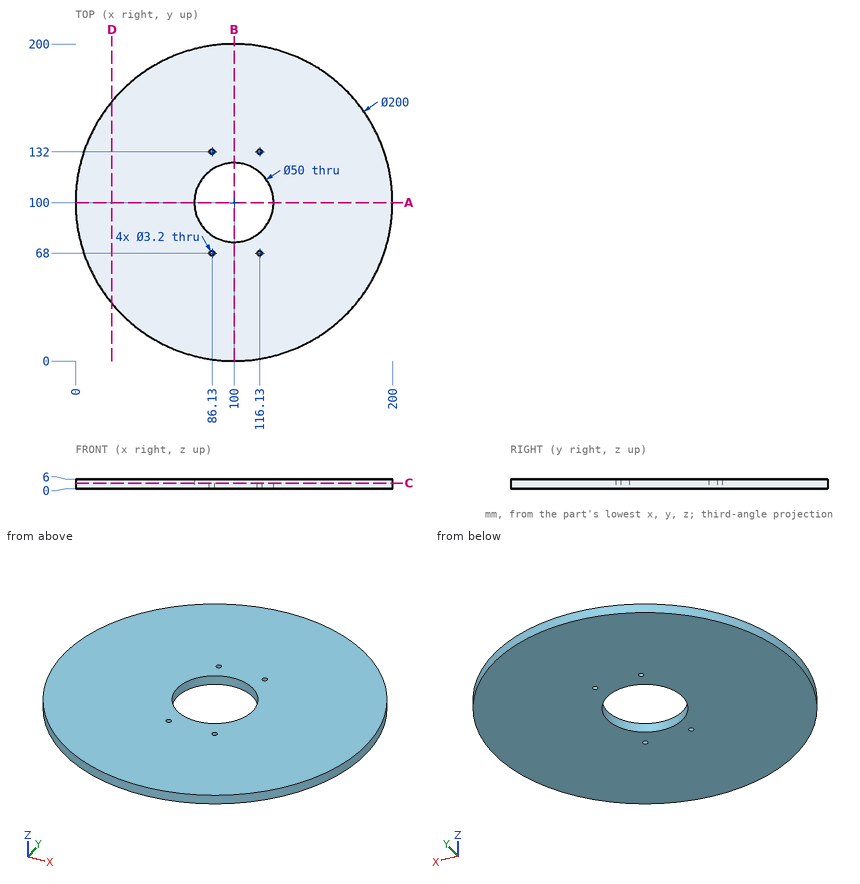
Print and shaded views of the part. All mm, measured from the part's lowest x, y and z. Give positions to 0.01 mm unless a question says otherwise; leave off trailing zeros. Write each loop counter-clockwise with the first axis right and the second up, starting at its lowest first coordinate (ties: lowest second). Pieces come first, ordered by that corner, then holes. Notation, with made-up numbers: (-22.75, -32.75) -> (-14.75, -32.75) arc R25 ccw to (-14.75, 1.25) -> close; hole circle Ø8 at (-15, 68.25). An arc over 180 degrees is marked (long way). Write item = value, one per line.
(1) Slice it at C-C, the plane z = 3.45. Give the cut face in (x, y).
Determined:
outline = circle Ø200 at (100, 100); hole circle Ø50 at (100, 100); hole circle Ø3.2 at (86.13, 68); hole circle Ø3.2 at (86.13, 132); hole circle Ø3.2 at (116.13, 68); hole circle Ø3.2 at (116.13, 132)
(2) Flat gauge pins, fed straight in: P1, Ø3, axis at y = 154, z = 5, coming from the -X side; P2, Ø3, axis at x = 142, z = 3.5, coming from the -Y side; P3, Ø3, axis at x = 73.5, z = 5, coming from the +Y side (1 decimal). Where does each tip first touch, or does it go through?
Determined:
P1 = 14.89
P2 = 8.57
P3 = 196.8
(3) Slice it at A-A, the plane y = 100. Give the cut face in (x, z), then the cut area to 3 significant figures.
Determined:
outline = (0, 0) -> (75, 0) -> (75, 6) -> (0, 6) -> close; (125, 0) -> (200, 0) -> (200, 6) -> (125, 6) -> close
area = 900 mm2
(4) Slice it at D-D, the plane x = 23. Give the cut face in (y, z).
Determined:
outline = (36.2, 0) -> (163.8, 0) -> (163.8, 6) -> (36.2, 6) -> close
(5) Probe line 1 along Y through (x, z) = (100, 3.15); line 2 along X through (y, z) = (132, 4.45); line 3 along X through (y, z) = (88, 3.65). List the from-to ranges inside material, lowest first.
Determined:
line_1 = 0 to 75, 125 to 200
line_2 = 5.26 to 84.53, 87.73 to 114.53, 117.73 to 194.74
line_3 = 0.72 to 78.07, 121.93 to 199.28
